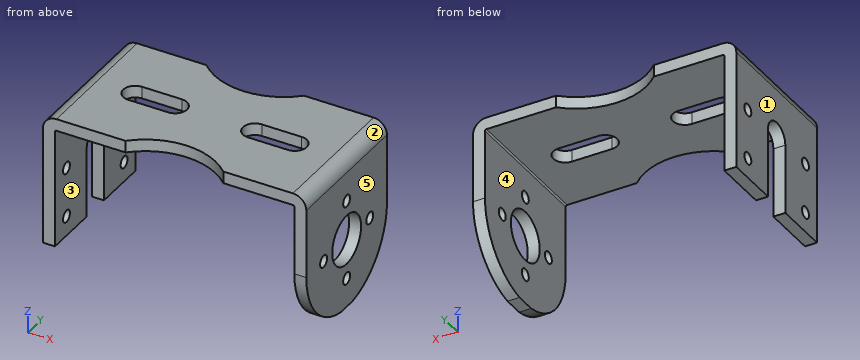
```python
from build123d import *

# Parameters (mm, degrees)
BASE_FLANGE1_DEPTH = 70
CUT_EXTRUDE1_DEPTH = 10
CUT_EXTRUDE3_START = -6
CUT_EXTRUDE3_DEPTH = 6
SKETCH8_R          = 12.5
SKETCH8_R_2        = 3
CUT_EXTRUDE4_DEPTH = 10
CUT_EXTRUDE6_DEPTH = 10
SKETCH12_R         = 3
CUT_EXTRUDE7_DEPTH = 10


# Read off the part's stored shape, not the designer's step: Cut-Extrude3
# Sheet-metal steps are written as plain solids
with BuildPart() as part:
    # Sketch1 → Base-Flange1 (new body)
    with BuildSketch(Plane(origin=(0, 0, 0), x_dir=(1, 0, 0), z_dir=(0, 1, 0))):
        with BuildLine():
            Line((0, 60), (0, 0.7366))
            ThreePointArc((0, 0.7366), (0.215745145, 0.215745145), (0.7366, 0))
            Line((0.7366, 0), (119.2634, 0))
            ThreePointArc((119.2634, 0), (119.784254855, 0.215745145), (120, 0.7366))
            Line((120, 0.7366), (120, 70))
            Line((120, 70), (126, 70))
            Line((126, 70), (126, 0.7366))
            ThreePointArc((126, 0.7366), (124.026895542, -4.026895542), (119.2634, -6))
            Line((119.2634, -6), (0.7366, -6))
            ThreePointArc((0.7366, -6), (-4.026895542, -4.026895542), (-6, 0.7366))
            Line((-6, 0.7366), (-6, 60))
            Line((-6, 60), (0, 60))
        make_face()
    extrude(amount=BASE_FLANGE1_DEPTH)

    # Sketch6 → Cut-Extrude1 (cut)
    with BuildSketch(Plane.XY.offset(6)):
        with BuildLine():
            Line((40, 29), (20, 29))
            ThreePointArc((20, 29), (14, 35), (20, 41))
            Line((20, 41), (40, 41))
            ThreePointArc((40, 41), (46, 35), (40, 29))
        make_face()
        with BuildLine():
            Line((80, 41), (100, 41))
            ThreePointArc((100, 41), (106, 35), (100, 29))
            Line((100, 29), (80, 29))
            ThreePointArc((80, 29), (74, 35), (80, 41))
        make_face()
    extrude(amount=-CUT_EXTRUDE1_DEPTH, mode=Mode.SUBTRACT)

    # Cut-Extrude3 outline → Cut-Extrude3 (cut)
    with BuildSketch(Plane(origin=(126, 0, 0), x_dir=(0, 0, -1), z_dir=(1, 0, 0)).offset(CUT_EXTRUDE3_START)):
        with BuildLine():
            Line((70, 0), (70, 29.935875682))
            ThreePointArc((70, 29.935875682), (58.256677497, 8.521288257), (35.3683, 0))
            Line((35.3683, 0), (70, 0))
        make_face()
        with BuildLine():
            ThreePointArc((35.3683, 70), (58.256677497, 61.478711743), (70, 40.064124318))
            Line((70, 40.064124318), (70, 70))
            Line((70, 70), (35.3683, 70))
        make_face()
    extrude(amount=CUT_EXTRUDE3_DEPTH, mode=Mode.SUBTRACT)

    # Sketch8 → Cut-Extrude4 (cut)
    with BuildSketch(Plane(origin=(126, 0, 0), x_dir=(0, 0, -1), z_dir=(1, 0, 0))):
        with Locations((35.3683, 35)):
            Circle(SKETCH8_R)
        with Locations((35.3683, 55)):
            Circle(SKETCH8_R_2)
        with Locations((55.3683, 35)):
            Circle(SKETCH8_R_2)
        with Locations((35.3683, 15)):
            Circle(SKETCH8_R_2)
        with Locations((15.3683, 35)):
            Circle(SKETCH8_R_2)
    extrude(amount=-CUT_EXTRUDE4_DEPTH, mode=Mode.SUBTRACT)

    # Sketch9 → Cut-Extrude6 (cut)
    with BuildSketch(Plane(origin=(0, 0, 0), x_dir=(-1, 0, 0), z_dir=(0, 0, -1))):
        with BuildLine():
            Line((-84.363131417, 70), (-35.373336561, 70))
            ThreePointArc((-35.373336561, 70), (-59.868233989, 60), (-84.363131417, 70))
        make_face()
        with BuildLine():
            Line((-84.363131417, 0), (-35.373336561, 0))
            ThreePointArc((-35.373336561, 0), (-59.868233989, 10), (-84.363131417, 0))
        make_face()
    extrude(amount=-CUT_EXTRUDE6_DEPTH, mode=Mode.SUBTRACT)

    # Sketch12 → Cut-Extrude7 (cut)
    with BuildSketch(Plane.ZY.offset(6)):
        with Locations((-50, 60)):
            Circle(SKETCH12_R)
        with Locations(Location((-25, 60, 0), (0, 0, 180))):
            Circle(SKETCH12_R)
        with Locations((-25, 10)):
            Circle(SKETCH12_R)
        with Locations(Location((-50, 10, 0), (0, 0, 180))):
            Circle(SKETCH12_R)
        with BuildLine():
            Line((-60, 42.5), (-25, 42.5))
            ThreePointArc((-25, 42.5), (-17.5, 35), (-25, 27.5))
            Line((-25, 27.5), (-60, 27.5))
            Line((-60, 27.5), (-60, 42.5))
        make_face()
    extrude(amount=-CUT_EXTRUDE7_DEPTH, mode=Mode.SUBTRACT)


solid = part.part
```
The listing builds one solid part. Answer for the finished solid, in the listing's coordinates (mm). Face numbers are marked on the shaded views. A direction names the side the tool comes from. Coordinates: 2 decimals unless noted, no trailing zeros. Loops run counter-clockwise (first coordinate to the right, second up) from the corner with the lowest first, then second, coordinate; pieces in that order, holes last. Notation, with made-up numbers: (-37.75, 27.5) - (-25.75, 27.5) arc R23 ccw to (-25.75, 42.5) - close; hole circle Ø3 at (-22, -0.75). An arc over 180 degrees is marked (long way). Use a Markdown table: item, result. Add a question column.
1) The part is cut by section A-A, the plane z = -6. Give the vertices of the cut face in (x, y), and give its area (3 significant figures).
2) Find the intervals of material crossed by line 1 (Y direction, x = -1.6, z = -25); line 2 (X direction, y = 60, z = -1); line 3 (X direction, y = 4, z = 1), in increasing order.
3) The part is cut by section C-C, the plane y = 55. Give the vertices of the cut face in (x, z), and give its area (3 significant figures).
4) The part is cut by section D-D, the plane x = 68.5. Give the vertices of the cut face in (y, z), and give its area (3 significant figures).
5) The part is cut by section B-B, the plane x = 31. Give the vertices of the cut face in (y, z).
6) Given pin 1 (3 mm diameter, centred on x = 61.5, y = 16, fed in from -Z); pin 2 (6.5 mm diameter, centred on x = 29, z = 2.5, fed in from -Y); pin 3 (5 mm diameter, centred on y = 10, z = -25, fed in from -X); pin 4 (6.5 mm diameter, centred on x = -2, y = 56.5, fed in from -Z), each flat-ended and moving along its own axis, determine where each tip first touches the part or whether it passes through.
7) The mould has two halves that part along X. Classify the marked faces 1, 2 and 3: released by +X, released by -X, zero draft, split by the parting line, or undercut.
8) For the marked faces 4 and 5, determine the directions among +Z, -Z, +X, -X, +Y, -Y from which every point of the face is accessible in a straight line to the end or side of a thin tool.
Here are the results:
| question | item | result |
|---|---|---|
| 1 | outline | (-6, 0) - (0, 0) - (0, 70) - (-6, 70) - close; (120, 0) - (126, 0) - (126, 70) - (120, 70) - close |
| 1 | area | 840 mm^2 |
| 2 | line 1 | y = 0 to 7, 13 to 27.5, 42.5 to 57, 63 to 70 |
| 2 | line 2 | x = -6 to 0, 120 to 126 |
| 2 | line 3 | x = -5.77 to 40.27, 79.46 to 125.77 |
| 3 | outline | (-6, -60) - (0, -60) - (0, -0.74) arc R0.74 cw to (0.74, 0) - (119.26, 0) arc R0.74 cw to (120, -0.74) - (120, -32.37) - (126, -32.37) - (126, -0.74) arc R6.74 ccw to (119.26, 6) - (0.74, 6) arc R6.74 ccw to (-6, -0.74) - close; (120, -64.09) - (126, -64.09) - (126, -38.37) - (120, -38.37) - close |
| 3 | area | 1,480 mm^2 |
| 4 | outline | (8.92, 0) - (61.08, 0) - (61.08, 6) - (8.92, 6) - close |
| 4 | area | 313 mm^2 |
| 5 | outline | (0, 0) - (29, 0) - (29, 6) - (0, 6) - close; (41, 0) - (70, 0) - (70, 6) - (41, 6) - close |
| 6 | pin 1 | stops at z = 0 |
| 6 | pin 2 | stops at y = 0 |
| 6 | pin 3 | stops at x = 120 |
| 6 | pin 4 | stops at z = -60 |
| 7 | face 1 | released by -X |
| 7 | face 2 | released by +X |
| 7 | face 3 | undercut |
| 8 | face 4 | -Z, +Y, -Y |
| 8 | face 5 | +Z, -Z, +X, +Y, -Y |
